```python
from build123d import *

# Parameters (mm, degrees)
F0_R     = 19.05
F1_DEPTH = 9.525
F2_R     = 2.54
F4_R     = 25.4
F4_R_2   = 16.26902
F5_DEPTH = 3.175
F6_R     = 12.784879
F7_DEPTH = 12.7


with BuildPart() as f1:
    # F0 (on Top) → F1 (new body)
    with BuildSketch(Plane.XY):
        with BuildLine():
            Line((-83.518586, -4.7625), (49.272146, -4.7625))
            ThreePointArc((49.272146, -4.7625), (99.621666, 0), (49.272146, 4.7625))
            Line((49.272146, 4.7625), (-83.518586, 4.7625))
            Line((-83.518586, 4.7625), (-80.384782, 42.441457))
            Line((-80.384782, 42.441457), (-86.286046, 42.932272))
            Line((-86.286046, 42.932272), (-89.460671, 4.7625))
            Line((-89.460671, 4.7625), (-103.127854, 4.7625))
            Line((-103.127854, 4.7625), (-103.127854, -4.7625))
            Line((-103.127854, -4.7625), (-89.460671, -4.7625))
            Line((-89.460671, -4.7625), (-86.286046, -42.932272))
            Line((-86.286046, -42.932272), (-80.384782, -42.441457))
            Line((-80.384782, -42.441457), (-83.518586, -4.7625))
        make_face()
        with Locations((74.221666, 0)):
            Circle(F0_R, mode=Mode.SUBTRACT)
    extrude(amount=F1_DEPTH)

    # F2
    f2_edges = [f1.edges().sort_by_distance(p)[0] for p in [
        (-17.12322, -4.7625, 9.525),
        (99.621666, 0, 9.525),
        (-17.12322, 4.7625, 9.525),
        (-81.951684, 23.601978, 9.525),
        (-83.335414, 42.686864, 9.525),
        (-87.873358, 23.847386, 9.525),
        (-96.294263, 4.7625, 9.525),
        (-103.127854, 0, 9.525),
        (-96.294263, -4.7625, 9.525),
        (-87.873358, -23.847386, 9.525),
        (-83.335414, -42.686864, 9.525),
        (-81.951684, -23.601978, 9.525),
        (55.171666, 0, 9.525),
        (-17.12322, -4.7625, 0),
        (99.621666, 0, 0),
        (-17.12322, 4.7625, 0),
        (-81.951684, 23.601978, 0),
        (-83.335414, 42.686864, 0),
        (-87.873358, 23.847386, 0),
        (-96.294263, 4.7625, 0),
        (-103.127854, 0, 0),
        (-96.294263, -4.7625, 0),
        (-87.873358, -23.847386, 0),
        (-83.335414, -42.686864, 0),
        (-81.951684, -23.601978, 0),
        (55.171666, 0, 0),
    ]]
    fillet(f2_edges, radius=F2_R)

    # F4 (on offset) → F5 (join)
    with BuildSketch(Plane.YZ.offset(25.4)):
        with Locations((0, 4.989178)):
            Circle(F4_R)
        with Locations((0, 4.989178)):
            Circle(F4_R_2, mode=Mode.SUBTRACT)
        with Locations((0, 4.989178)):
            Circle(F4_R_2)
    extrude(amount=F5_DEPTH)

    # F6 (on face) → F7 (join)
    with BuildSketch(Plane.YZ.offset(28.575)):
        with Locations((0, 4.989178)):
            Circle(F6_R)
        with BuildLine():
            ThreePointArc((-2.2225, 0), (-4.018551, 0.743949), (-4.7625, 2.54))
            Line((-4.7625, 2.54), (-4.7625, 6.985))
            ThreePointArc((-4.7625, 6.985), (-4.018551, 8.781051), (-2.2225, 9.525))
            Line((-2.2225, 9.525), (2.2225, 9.525))
            ThreePointArc((2.2225, 9.525), (4.018551, 8.781051), (4.7625, 6.985))
            Line((4.7625, 6.985), (4.7625, 2.54))
            ThreePointArc((4.7625, 2.54), (4.018551, 0.743949), (2.2225, 0))
            Line((2.2225, 0), (-2.2225, 0))
        make_face(mode=Mode.SUBTRACT)
    extrude(amount=F7_DEPTH)


solid = f1.part
```
Can you work these out from the model? Positions are in its coordinate system, mm. A direction names the side the tool comes from. Coordinates: 2 decimals unless noted, no trailing zeros. Order: outer loops, then holes, each group sorted by start corner. A loop starts at its lowest first (then second) coordinate and runs counter-clockwise, first axis right, second up. Notation, with made-up numbers: (4.25, 34.25) - (14.25, 34.25) arc R8 cw to (14.25, 45.25) - close; hole circle Ø8 at (77.5, -16). An arc over 180 degrees is marked (long way). Answer in a Markdown table with one row per item.
1. Suppose I cut it at A-A (y = 0). Please give me the cut outline in (x, z) (3 decimals).
Reply:
| item | result |
|---|---|
| outline | (-103.128, 2.54) arc R2.54 ccw to (-100.588, 0) - (25.4, 0) - (25.4, -20.411) - (28.575, -20.411) - (28.575, -7.796) - (41.275, -7.796) - (41.275, 0) - (52.632, 0) arc R2.54 ccw to (55.172, 2.54) - (55.172, 6.985) arc R2.54 ccw to (52.632, 9.525) - (41.275, 9.525) - (41.275, 17.774) - (28.575, 17.774) - (28.575, 30.389) - (25.4, 30.389) - (25.4, 9.525) - (-100.588, 9.525) arc R2.54 ccw to (-103.128, 6.985) - close; (93.272, 2.54) arc R2.54 ccw to (95.812, 0) - (97.082, 0) arc R2.54 ccw to (99.622, 2.54) - (99.622, 6.985) arc R2.54 ccw to (97.082, 9.525) - (95.812, 9.525) arc R2.54 ccw to (93.272, 6.985) - close |
2. If we mould it in two halves opening along X, with no side actions, what happens to faces 5 (the cylindrical face through (-82.764, 22.57, 0.764)), 6 (the flat face through (-96, -4.762, 5)), 7 (the cylindrical face through (-87.27, 22.34, 0.76))? For each: pulls with the +X half, pulls with the -X half, needs draft (parallel to the pull), parting line crosses it, or undercut.
Reply:
| item | result |
|---|---|
| face 5 | undercut |
| face 6 | needs draft |
| face 7 | pulls with the -X half |
3. Suppose I cut it at D-D (z = 23). Please give me the cut outline in (x, y) (3 decimals), and give its area (3 significant figures).
Reply:
| item | result |
|---|---|
| outline | (25.4, -17.91) - (28.575, -17.91) - (28.575, 17.91) - (25.4, 17.91) - close |
| area | 114 mm^2 |
4. For faces 1 (the flat face through (52.5, 1.8, 0)), 2 (the flat face through (-96, 4.762, 5)), 3 (the flat face through (41.275, 0, -1)), 4 (the cylindrical face through (-82.811, -22.004, 0.764)), which set-ups out of +Z, -Z, +X, -X, +Y, -Y let a thin tool reach every point of the face, with its end or its side?
Reply:
| item | result |
|---|---|
| face 1 | -Z, +X, +Y, -Y |
| face 2 | +Z, -Z, -X, +Y |
| face 3 | none |
| face 4 | -Z |
5. Suppose I cut it at C-C (z = -3). Please give me the cut outline in (x, y) (3 decimals), and give its area (3 significant figures).
Reply:
| item | result |
|---|---|
| outline | (25.4, -24.111) - (28.575, -24.111) - (28.575, -9.981) - (41.275, -9.981) - (41.275, 9.981) - (28.575, 9.981) - (28.575, 24.111) - (25.4, 24.111) - close |
| area | 407 mm^2 |
6. Suppose I cut it at B-B (x = -40). Please give me the cut outline in (y, z) (1 decimal), and give its area (3 significant figures).
Reply:
| item | result |
|---|---|
| outline | (-4.8, 2.5) arc R2.5 ccw to (-2.2, 0) - (2.2, 0) arc R2.5 ccw to (4.8, 2.5) - (4.8, 7) arc R2.5 ccw to (2.2, 9.5) - (-2.2, 9.5) arc R2.5 ccw to (-4.8, 7) - close |
| area | 85.2 mm^2 |
7. For pin 1 (1.3 mm diameter, centred on x = 43.5, z = 3.5, fed in from -Y); pin 2 (24 mm diameter, centred on x = -23.5, y = -2, fed in from +Z) (3 decimals); pin 3 (12 mm diameter, centred on x = 7.5, z = 2.5, fed in from +Y), each with a flat end and sliding along its axis, tell me the tip position at first contact or that it passes through.
Reply:
| item | result |
|---|---|
| pin 1 | stops at y = -4.76 |
| pin 2 | stops at z = 9.525 |
| pin 3 | stops at y = 4.76 |
8. If I drill on line 1 along Y through (x, z) = (43, 5); line 2 along Y through (x, z) = (78.5, 5); line 3 along X through (y, z) = (1, -8) (3 decimals), over which ranges is the centre line in solid material (lowest first)?
Reply:
| item | result |
|---|---|
| line 1 | y = -4.76 to 4.76 |
| line 2 | y = -25.04 to -18.56, 18.56 to 25.04 |
| line 3 | x = 25.4 to 28.575 |
